from build123d import *

# Parameters (mm, degrees)
SKETCH001_R       = 45
PAD_DEPTH         = 1
PAD003_DEPTH      = 31
PAD003_DEPTH_BACK = 1
PAD004_DEPTH      = 31
PAD004_DEPTH_BACK = 1
SKETCH026_R       = 11.2
POCKET_DEPTH      = 169.3567157682
SKETCH027_R       = 11.2
POCKET001_DEPTH   = 207.6737429392


with BuildPart() as part:
    # Sketch001 → Pad (new body)
    with BuildSketch(Plane.XY):
        with BuildLine():
            Line((50, 74), (0, 74))
            ThreePointArc((0, 74), (-74.0000001202, 0), (0, -74))
            Line((73, 0), (0, -74))
            Line((73, 51), (73, 0))
            ThreePointArc((73, 51), (66.2634559673, 67.2634559673), (50, 74))
        make_face()
        Circle(SKETCH001_R, mode=Mode.SUBTRACT)
    extrude(amount=-PAD_DEPTH)

    # Sketch → Pad003 (new body, two sides)
    with BuildSketch(Plane.XY) as pad003_sk:
        Polygon((22.252644507, 72.2162499408), (64.4702727046, 72.2162499408), (67.8254301255, 77.1904753762), (38.809115086, 96.7622269976), align=None)
    extrude(amount=PAD003_DEPTH)
    extrude(pad003_sk.sketch, amount=-PAD003_DEPTH_BACK)

    # Sketch025 → Pad004 (new body, two sides)
    with BuildSketch(Plane.XY) as pad004_sk:
        Polygon((-69.1718947306, 40.2246535265), (-79.4049043959, 6.7539870678), (-73.6670758601, 4.9997568394), (-63.4340661948, 38.4704232981), align=None)
    extrude(amount=PAD004_DEPTH)
    extrude(pad004_sk.sketch, amount=-PAD004_DEPTH_BACK)

    # Sketch026 → Pocket (cut, through all)
    with BuildSketch(Plane(origin=(-74.5056676119, 22.7786685315, 0), x_dir=(-0.2923717047, -0.956304756, 0), z_dir=(-0.956304756, 0.2923717047, 0))):
        with Locations((-0.743122693, 31)):
            Circle(SKETCH026_R)
    extrude(amount=-POCKET_DEPTH, mode=Mode.SUBTRACT)

    # Sketch027 → Pocket001 (cut, through all)
    with BuildSketch(Plane(origin=(56.9936696471, 84.4965900712, 0), x_dir=(-0.8290375726, 0.5591929035, 0), z_dir=(0.5591929035, 0.8290375726, 0))):
        with Locations((4.4345360972, 31)):
            Circle(SKETCH027_R)
    extrude(amount=-POCKET001_DEPTH, mode=Mode.SUBTRACT)


solid = part.part
Check sheet for the modelled part. Datum: model origin and axes. Units: mm. Round coordinates to 2 decimals unless told otherwise and drop trailing zeros. Write each loop counter-clockwise with the first axis right and the second up, starting at its lowest first coordinate (ties: lowest second). Pieces come first, ordered by that corner, then holes. Notation, with made-up numbers: (45.25, 12) - (74.25, 12) arc R28 ccw to (74.25, 47) - close; hole circle Ø1 at (-23.75, 1). An arc over 180 degrees is marked (long way). Return JSON: item names as keys, results as strings.
Q1. Scan lines: L1, parallel to Y at x = 0, z = -0.7; L2, parallel to Z at x = -62, y = -8.5; L3, parallel to Y at x = 28, z = 3.5. Record each from-to range of solid material in increasing order. Write a range as from..to.
Returned:
{"L1": "y = -74..-45, 45..74", "L2": "z = -1..0", "L3": "y = 72.22..80.74"}
Q2. Cross-section at A-A (z = 24.5). Record the boundary of the cut face in (x, y), then the cut area to 3 significant figures.
Returned:
{"outline": "(-79.4, 6.75) - (-73.67, 5) - (-71.22, 13.01) - (-76.96, 14.77) - close; (-71.62, 32.21) - (-65.88, 30.46) - (-63.43, 38.47) - (-69.17, 40.22) - close; (22.25, 72.22) - (32.36, 72.22) - (45.76, 92.08) - (38.81, 96.76) - close; (54.36, 72.22) - (64.47, 72.22) - (67.83, 77.19) - (60.88, 81.88) - close", "area": "399 mm²"}
Q3. Cross-section at B-B (x = 5). Record the boundary of the cut face in (y, z).
Returned:
{"outline": "(-68.93, -1) - (-44.72, -1) - (-44.72, 0) - (-68.93, 0) - close; (44.72, -1) - (74, -1) - (74, 0) - (44.72, 0) - close"}
Q4. Draft check along Y on faces 1 (the flat face through (-66.263, 39.335, 15.224)), 2 (the cylindrical face through (20.765, -39.923, -0.493)), 3 (the flat face through (62, 76, 31)). Enter one of: released by +Y, released by -Y, zero draft, split by the parting line, or undercut.
Returned:
{"face 1": "released by +Y", "face 2": "undercut", "face 3": "zero draft"}
Q5. Depth check by flat-ended pin: P1, Ø1.5, axis at x = -59.5, y = -44.5, coming from the +Z side; P2, Ø1.1, axis at x = 16.5, z = -0.5, coming from the +Y side; P3, Ø3, axis at y = 13, z = 25, coming from the -X side. Enter the tip coordinate at first touch or a pass-through.
Returned:
{"P1": "stops at z = 0", "P2": "stops at y = 74", "P3": "stops at x = -77.95"}
Q6. Cross-section at C-C (z = 12). Record the boundary of the cut face in (x, y).
Returned:
{"outline": "(-79.4, 6.75) - (-73.67, 5) - (-63.43, 38.47) - (-69.17, 40.22) - close; (22.25, 72.22) - (64.47, 72.22) - (67.83, 77.19) - (38.81, 96.76) - close"}
Q7. Cross-section at D-D (x = 27). Record the boundary of the cut face in (y, z), then the cut area to 3 significant figures.
Returned:
{"outline": "(-46.63, -1) - (-36, -1) - (-36, 0) - (-46.63, 0) - close; (36, -1) - (79.25, -1) - (79.25, 31) - (72.22, 31) - (72.22, 0) - (36, 0) - close", "area": "272 mm²"}
